CAD build for the part. Positions are in the model's coordinates, mm. Face numbers are marked on the shaded views. A direction names the side the tool comes from. Give positions to 0.01 mm unless a question says otherwise; leave off trailing zeros. Order: outer loops, then holes, each group sorted by start corner. A loop starts at its lowest first (then second) coordinate and runs counter-clockwise, first axis right, second up. Notation, with made-up numbers: (58.5, -2.75) -> (72.5, -2.75) arc R30 cw to (72.5, 36.25) -> close; hole circle Ø2 at (-32, -3). An arc over 180 degrees is marked (long way). Answer as CSV lines item,"result".
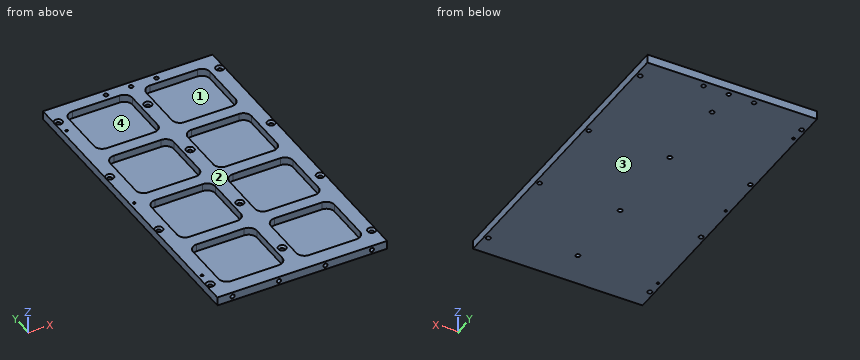
```python
from build123d import *

# Parameters (mm, degrees)
SKETCH_W            = 168
SKETCH_H            = 309
PAD_DEPTH           = 8.5
POCKET_DEPTH        = 7.5
HOLE_D              = 4.4
HOLE_DEPTH          = 25
HOLE_CSINK_D        = 8
HOLE_CSINK_ANGLE    = 90
HOLE001_D           = 4.4
HOLE001_DEPTH       = 25
HOLE001_CSINK_D     = 8
HOLE001_CSINK_ANGLE = 90
SKETCH003_R         = 2.05
HOLE002_DEPTH       = 10.768236
HOLE002_TIPS_R      = 2.05
SKETCH005_R         = 2.05
HOLE003_DEPTH       = 8.501
SKETCH006_R         = 1.25
HOLE004_DEPTH       = 25


with BuildPart() as part:
    # Sketch → Pad (new body)
    with BuildSketch(Plane.XY):
        Rectangle(SKETCH_W, SKETCH_H)
    extrude(amount=-PAD_DEPTH)

    # Sketch001 → Pocket (cut)
    with BuildSketch(Plane.XY):
        with BuildLine():
            Line((-62, -78.5), (-15, -78.5))
            ThreePointArc((-7, -86.5), (-9.343146, -80.843146), (-15, -78.5))
            Line((-7, -86.5), (-7, -131.5))
            ThreePointArc((-15, -139.5), (-9.343146, -137.156854), (-7, -131.5))
            Line((-15, -139.5), (-62, -139.5))
            ThreePointArc((-70, -131.5), (-67.656854, -137.156854), (-62, -139.5))
            Line((-70, -131.5), (-70, -86.5))
            ThreePointArc((-62, -78.5), (-67.656854, -80.843146), (-70, -86.5))
        make_face()
        with BuildLine():
            Line((15, -78.5), (62, -78.5))
            ThreePointArc((70, -86.5), (67.656854, -80.843146), (62, -78.5))
            Line((70, -86.5), (70, -131.5))
            ThreePointArc((62, -139.5), (67.656854, -137.156854), (70, -131.5))
            Line((62, -139.5), (15, -139.5))
            ThreePointArc((7, -131.5), (9.343146, -137.156854), (15, -139.5))
            Line((7, -131.5), (7, -86.5))
            ThreePointArc((15, -78.5), (9.343146, -80.843146), (7, -86.5))
        make_face()
        with BuildLine():
            Line((-62, -5), (-15, -5))
            ThreePointArc((-7, -13), (-9.343146, -7.343146), (-15, -5))
            Line((-7, -13), (-7, -58))
            ThreePointArc((-15, -66), (-9.343146, -63.656854), (-7, -58))
            Line((-15, -66), (-62, -66))
            ThreePointArc((-70, -58), (-67.656854, -63.656854), (-62, -66))
            Line((-70, -58), (-70, -13))
            ThreePointArc((-62, -5), (-67.656854, -7.343146), (-70, -13))
        make_face()
        with BuildLine():
            Line((15, -5), (62, -5))
            ThreePointArc((70, -13), (67.656854, -7.343146), (62, -5))
            Line((70, -13), (70, -58))
            ThreePointArc((62, -66), (67.656854, -63.656854), (70, -58))
            Line((62, -66), (15, -66))
            ThreePointArc((7, -58), (9.343146, -63.656854), (15, -66))
            Line((7, -58), (7, -13))
            ThreePointArc((15, -5), (9.343146, -7.343146), (7, -13))
        make_face()
        with BuildLine():
            Line((-62, 68.5), (-15, 68.5))
            ThreePointArc((-7, 60.5), (-9.343146, 66.156854), (-15, 68.5))
            Line((-7, 60.5), (-7, 15.5))
            ThreePointArc((-15, 7.5), (-9.343146, 9.843146), (-7, 15.5))
            Line((-15, 7.5), (-62, 7.5))
            ThreePointArc((-70, 15.5), (-67.656854, 9.843146), (-62, 7.5))
            Line((-70, 15.5), (-70, 60.5))
            ThreePointArc((-62, 68.5), (-67.656854, 66.156854), (-70, 60.5))
        make_face()
        with BuildLine():
            Line((15, 68.5), (62, 68.5))
            ThreePointArc((70, 60.5), (67.656854, 66.156854), (62, 68.5))
            Line((70, 60.5), (70, 15.5))
            ThreePointArc((62, 7.5), (67.656854, 9.843146), (70, 15.5))
            Line((62, 7.5), (15, 7.5))
            ThreePointArc((7, 15.5), (9.343146, 9.843146), (15, 7.5))
            Line((7, 15.5), (7, 60.5))
            ThreePointArc((15, 68.5), (9.343146, 66.156854), (7, 60.5))
        make_face()
        with BuildLine():
            Line((-62, 142), (-15, 142))
            ThreePointArc((-7, 134), (-9.343146, 139.656854), (-15, 142))
            Line((-7, 134), (-7, 89))
            ThreePointArc((-15, 81), (-9.343146, 83.343146), (-7, 89))
            Line((-15, 81), (-62, 81))
            ThreePointArc((-70, 89), (-67.656854, 83.343146), (-62, 81))
            Line((-70, 89), (-70, 134))
            ThreePointArc((-62, 142), (-67.656854, 139.656854), (-70, 134))
        make_face()
        with BuildLine():
            Line((15, 142), (62, 142))
            ThreePointArc((70, 134), (67.656854, 139.656854), (62, 142))
            Line((70, 134), (70, 89))
            ThreePointArc((62, 81), (67.656854, 83.343146), (70, 89))
            Line((62, 81), (15, 81))
            ThreePointArc((7, 89), (9.343146, 83.343146), (15, 81))
            Line((7, 89), (7, 134))
            ThreePointArc((15, 142), (9.343146, 139.656854), (7, 134))
        make_face()
    extrude(amount=-POCKET_DEPTH, mode=Mode.SUBTRACT)

    # Hole
    with Locations(Plane.XY):
        with Locations((80, 134.5), (80, 43.5), (80, -43.5), (80, -134.5)):
            hole = CounterSinkHole(HOLE_D / 2, HOLE_CSINK_D / 2, depth=HOLE_DEPTH, counter_sink_angle=HOLE_CSINK_ANGLE)

    # Mirrored: Hole across Sketch002 V_Axis
    add(hole.mirror(Plane(origin=(0, 0, 0), x_dir=(0, 0, 1), z_dir=(1, 0, 0))), mode=Mode.SUBTRACT)

    # Hole001
    with Locations(Plane.XY):
        with Locations((0, 119), (0, 44), (0, -44), (0, -119)):
            CounterSinkHole(HOLE001_D / 2, HOLE001_CSINK_D / 2, depth=HOLE001_DEPTH, counter_sink_angle=HOLE001_CSINK_ANGLE)

    # Sketch003 (on DatumPlane) → Hole002 (cut)
    with BuildSketch(Plane.XZ.offset(154.5)):
        with Locations((-69, -4.25)):
            Circle(SKETCH003_R)
        with Locations((-23, -4.25)):
            Circle(SKETCH003_R)
        with Locations((23, -4.25)):
            Circle(SKETCH003_R)
        with Locations((69, -4.25)):
            Circle(SKETCH003_R)
    extrude(amount=-HOLE002_DEPTH, mode=Mode.SUBTRACT)

    # Hole002 tips → Hole002 tip 1 section 0
    with BuildSketch(Plane.XZ.offset(143.731764), mode=Mode.PRIVATE) as hole002_tip_1_s0:
        with Locations((-69, -4.25)):
            Circle(HOLE002_TIPS_R)
    loft([hole002_tip_1_s0.sketch, Vertex(-69, -142.5, -4.25)], mode=Mode.SUBTRACT)

    # Hole002 tips → Hole002 tip 2 section 0
    with BuildSketch(Plane.XZ.offset(143.731764), mode=Mode.PRIVATE) as hole002_tip_2_s0:
        with Locations((-23, -4.25)):
            Circle(HOLE002_TIPS_R)
    loft([hole002_tip_2_s0.sketch, Vertex(-23, -142.5, -4.25)], mode=Mode.SUBTRACT)

    # Hole002 tips → Hole002 tip 3 section 0
    with BuildSketch(Plane.XZ.offset(143.731764), mode=Mode.PRIVATE) as hole002_tip_3_s0:
        with Locations((23, -4.25)):
            Circle(HOLE002_TIPS_R)
    loft([hole002_tip_3_s0.sketch, Vertex(23, -142.5, -4.25)], mode=Mode.SUBTRACT)

    # Hole002 tips → Hole002 tip 4 section 0
    with BuildSketch(Plane.XZ.offset(143.731764), mode=Mode.PRIVATE) as hole002_tip_4_s0:
        with Locations((69, -4.25)):
            Circle(HOLE002_TIPS_R)
    loft([hole002_tip_4_s0.sketch, Vertex(69, -142.5, -4.25)], mode=Mode.SUBTRACT)

    # Sketch005 → Hole003 (cut, through all)
    with BuildSketch(Plane.XY):
        with Locations((25, 148.5)):
            Circle(SKETCH005_R)
        with Locations((0, 148.5)):
            Circle(SKETCH005_R)
        with Locations((-25, 148.5)):
            Circle(SKETCH005_R)
    extrude(amount=-HOLE003_DEPTH, mode=Mode.SUBTRACT)

    # Sketch006 → Hole004 (cut)
    with BuildSketch(Plane.XY):
        with Locations((-80, 120)):
            Circle(SKETCH006_R)
        with Locations((-80, 0)):
            Circle(SKETCH006_R)
        with Locations((-80, -120)):
            Circle(SKETCH006_R)
    extrude(amount=-HOLE004_DEPTH, mode=Mode.SUBTRACT)


solid = part.part
```
1) Band-saw the part on B-B, the plane y = -100. Write the cut outline in (x, z), then the cut area to 3 significant figures.
Data:
outline,"(-84, -8.5) -> (84, -8.5) -> (84, 0) -> (70, 0) -> (70, -7.5) -> (7, -7.5) -> (7, 0) -> (-7, 0) -> (-7, -7.5) -> (-70, -7.5) -> (-70, 0) -> (-84, 0) -> close"
area,"483 mm2"
2) Pull direction X, two halves, no side cores. Call the marked faces 1 and 2: pulls with the +X half, pulls with the -X half, needs draft (parallel to the pull), parting line crosses it, or undercut.
Data:
face 1,"undercut"
face 2,"needs draft"
3) Band-saw the part on A-A, the plane x = 45. Write the cut outline in (y, z).
Data:
outline,"(-154.5, -8.5) -> (154.5, -8.5) -> (154.5, 0) -> (142, 0) -> (142, -7.5) -> (81, -7.5) -> (81, 0) -> (68.5, 0) -> (68.5, -7.5) -> (7.5, -7.5) -> (7.5, 0) -> (-5, 0) -> (-5, -7.5) -> (-66, -7.5) -> (-66, 0) -> (-78.5, 0) -> (-78.5, -7.5) -> (-139.5, -7.5) -> (-139.5, 0) -> (-154.5, 0) -> close"
4) Pin check, flat tips, straight feed: P1, Ø4, axis at x = 12, y = 85.5, coming from the +Z side; P2, Ø5.5, axis at x = 0, y = -44, coming from the +Z side. Stop position of each tip, or through.
Data:
P1,"stops at z = -7.5"
P2,"stops at z = -1.25"
5) Wall check: line 1 along X through (y, z) = (46.5, -3.75); line 2 along Y through (x, z) = (-48.5, -4.25); line 3 along Y through (x, z) = (-63, -6.25). Give the ranges that are in metal, low to high. Write a range as [from, to].
Data:
line 1,"x = [-84, -70], [-7, 7], [70, 84]"
line 2,"y = [-154.5, -139.5], [-78.5, -66], [-5, 7.5], [68.5, 81], [142, 154.5]"
line 3,"y = [-154.5, -139.44], [-78.56, -65.94], [-5.06, 7.56], [68.44, 81.06], [141.94, 154.5]"
6) Which spindle directions (+Z, -Z, +X, -X, +Y, -Y) get a long thin tool onto all of the face, cutting with end or side? Do the marked faces 3 and 4. Say none if no direction does.
Data:
face 3,"-Z, +X, -X, +Y, -Y"
face 4,"+Z"
